Here's how the part is built. I have some questions about the finished solid (model axes, mm). A direction names the side the tool comes from. Give positions to 0.01 mm unless a question says otherwise; leave off trailing zeros. Write each loop counter-clockwise with the first axis right and the second up, starting at its lowest first coordinate (ties: lowest second). Pieces come first, ordered by that corner, then holes. Notation, with made-up numbers: (68, -1) -> (126, -1) arc R6 cw to (126, 7) -> close; hole circle Ø4 at (-7.75, 73.5). An arc over 180 degrees is marked (long way). Put each result on its own line as item: value. Start each with the question number.
Autodesk Inventor part; units mm, degrees
ref_plane "YZ Plane" through (0, 0, 0) normal (1, 0, 0) x (0, 1, 0)
ref_plane "XZ Plane" through (0, 0, 0) normal (0, 1, 0) x (-1, 0, 0)
ref_plane "XY Plane" through (0, 0, 0) normal (0, 0, 1) x (1, 0, 0)
sketch "Sketch1" plane through (0, 0, 0) normal (0, 1, 0) x (-1, 0, 0)
  circle A0 centre (0, 0) radius 52.9167
  circle A1 centre (0, 0) radius 72.39
  dimension "d0" = 105.8333
  dimension "d1" = 144.78
extrude "Extrusion1" add sketch "Sketch1" against normal blind 12.7
sketch "Sketch2" plane through (0, 0, 0) normal (0, 1, 0) x (1, 0, 0)
  circle A0 centre (0, 64.5584) radius 2.54
  point P0 (0, 0)
  dimension "d5" = 5.08
  dimension "d6" = 64.5584
extrude "Extrusion2" cut sketch "Sketch2" against normal through all
sketch "Sketch3" plane through (0, 0, 0) normal (0, 1, 0) x (1, 0, 0)
  circle A0 centre (0, 64.5584) radius 5.715
  point P0 (0, 0)
  dimension "d9" = 64.5584
  dimension "d10" = 11.43
extrude "Extrusion3" cut sketch "Sketch3" against normal blind 6.35
pattern_circular "Circular Pattern3" count 15 over 360 about axis through (0, 0, 0) along (0, -1, 0) of "Extrusion2", "Extrusion3"
properties part number "wormGearSupport"
1) I want a section at A-A, the plane x = 0. Write out the boundary of the cut face in (y, z), and give its area (3 significant figures).
2) I need wall thicknesses on probe 1 along Z at (x, y) = (-29, -1.75); probe 2 along Z at (x, y) = (-28.5, -5.5); probe 3 along X at (y, z) = (-0.5, -24). Which ranges of each line are inside material? Lowest first, please.
3) Which directions (+Z, -Z, +X, -X, +Y, -Y) give clear straight access to the entire face, cutting with the end or side of a thin tool? Please do faces 5 (the cylindrical face through (63.858, -9.481, -19.313)), 6 (the flat face through (10.8, -6.35, 62.5)).
4) I want a section at B-B, the plane z = 17.5. Write out the boundary of the cut face in (x, y).
5) Thinking about a two-plate mould opening in Z: for faces 1 (the flat face through (53.6, -6.35, 33.8)), 2 (the cylindrical face through (-32.233, -3.131, 52.081)), 3 (the flat face through (-21, 0, 49)), 4 (the cylindrical face through (57.446, -6.261, -44.048)), which applies, released by +Z, released by -Z, zero draft, split by the parting line, or undercut?
6) I'm going to push flat-ended pins straight in: pin 1 Ø9 at (x, z) = (-24, -56.5) entering from +Y; pin 2 Ø3 at (x, z) = (-61.4, -19.95) entering from +Y; pin 3 Ø7 at (x, z) = (-13.42, 63.15) entering from +Y; pin 4 Ø3 at (x, y) = (30, -7.5) entering from -Z. Where does each tip first touch, or does it pass through?
Established:
1. outline: (-12.7, -72.39) -> (0, -72.39) -> (0, -70.27) -> (-6.35, -70.27) -> (-6.35, -67.1) -> (-12.7, -67.1) -> close; (-12.7, -62.02) -> (-6.35, -62.02) -> (-6.35, -58.84) -> (0, -58.84) -> (0, -52.92) -> (-12.7, -52.92) -> close; (-12.7, 52.92) -> (0, 52.92) -> (0, 72.39) -> (-12.7, 72.39) -> close
1. area: 390 mm2
2. probe 1: z = -66.33 to -63.99, -53.96 to -44.26, 44.26 to 66.33
2. probe 2: z = -66.54 to -64.23, -53.72 to -44.59, 44.59 to 66.54
2. probe 3: x = -68.3 to -65.43, -57.37 to -47.16, 47.16 to 57.37, 65.43 to 68.3
3. face 5: +Y, -Y
3. face 6: +Y
4. outline: (-70.24, -12.7) -> (-49.94, -12.7) -> (-49.94, 0) -> (-70.24, 0) -> close; (49.94, -12.7) -> (70.24, -12.7) -> (70.24, 0) -> (49.94, 0) -> close
5. face 1: undercut
5. face 2: undercut
5. face 3: zero draft
5. face 4: split by the parting line
6. pin 1: stops at y = 0
6. pin 2: passes through
6. pin 3: stops at y = -6.35
6. pin 4: stops at z = -66.54
